CAD build for the part. Positions are in the model's coordinates, mm. Round coordinates to 2 decimals unless told otherwise and drop trailing zeros. Loops run counter-clockwise (first coordinate to the right, second up) from the corner with the lowest first, then second, coordinate; pieces in that order, holes last. Notation, with made-up numbers: (60.25, 50) -> (70.25, 50) arc R25 ccw to (70.25, 89) -> close; hole circle Ø10 at (8.5, 2.25). An arc over 180 degrees is marked (long way). Answer as CSV lines item,"result".
```python
from build123d import *

# Parameters (mm, degrees)
M2_5_TAPPED_HOLE1_D           = 2.05
M2_5_TAPPED_HOLE1_ON_FACE_2_D = 2.05


with BuildPart() as part:
    # Sketch1 → Revolve1 (revolve)
    with BuildSketch(Plane.XY, mode=Mode.PRIVATE) as revolve1_sk:
        Polygon((0, 7.5), (36.519586152, 14), (36.519586152, 16.526331), (-23.480413848, 16.526331), (-23.480413848, 12.526331), align=None)
    revolve(revolve1_sk.sketch.rotate(Axis((-21.926609295, 0, 0), (1, 0, 0)), 90), axis=Axis((-21.926609295, 0, 0), (1, 0, 0)))

    # M2.5 Tapped Hole1 (through all)
    with Locations(Plane(origin=(-20.480413848, 0, -16.526331), x_dir=(0, -1, 0), z_dir=(0, 0, -1))):
        with Locations((0, 0)):
            Hole(M2_5_TAPPED_HOLE1_D / 2)

    # M2.5 Tapped Hole1 on face 2 (through all)
    with Locations(Plane(origin=(-20.480413848, 16.526331, 0), x_dir=(0, 0, 1), z_dir=(0, 1, 0))):
        with Locations((0, 0)):
            Hole(M2_5_TAPPED_HOLE1_ON_FACE_2_D / 2)


solid = part.part
```
Q1. Slice it at D-D, the plane x = 9. Give the cut face in (y, z).
Results:
outline,"circle Ø33.05 at (0, 0); hole circle Ø18.2 at (0, 0)"
Q2. Probe L1, parallel to Z at x = 21.5, y = -3.5; L2, parallel to Z at x = -10.5, y = 6.5; L3, parallel to Y at x = -16, z = 5.5. List the from-to ranges inside material, lowest first. Write a range as [from, to].
Results:
L1,"[-16.15, -10.77], [10.77, 16.15]"
L2,"[-15.19, -7.26], [7.26, 15.19]"
L3,"[-15.58, -9.44], [9.44, 15.58]"
Q3. Slice it at A-A, the plane y = 0. Give the cut face in (x, z), and give its area (3 significant figures).
Results:
outline,"(-23.48, -16.53) -> (-21.51, -16.53) -> (-21.51, -12.1) -> (-23.48, -12.53) -> close; (-23.48, 12.53) -> (-21.51, 12.1) -> (-21.51, 16.53) -> (-23.48, 16.53) -> close; (-19.46, -16.53) -> (36.52, -16.53) -> (36.52, -14) -> (0, -7.5) -> (-19.46, -11.66) -> close; (-19.46, 11.66) -> (0, 7.5) -> (36.52, 14) -> (36.52, 16.53) -> (-19.46, 16.53) -> close"
area,"709 mm2"
Q4. Drop flat-ended pins along their axis: pin 1 Ø6 at (x, y) = (25, 13) entering from +Z; pin 2 Ø8 at (x, y) = (0.5, 5) entering from +Z; pin 3 Ø1 at (y, z) = (-3, 6) entering from +X; pin 4 Ø6 at (x, z) = (-6, -9.5) entering from +Y. Give the stop position or say it passes through.
Results:
pin 1,"z = 13.16"
pin 2,"z = 16.5"
pin 3,"through"
pin 4,"y = 15.19"
Q5. Slice it at C-C, the plane x = -8. Give the cut face in (y, z).
Results:
outline,"circle Ø33.05 at (0, 0); hole circle Ø18.43 at (0, 0)"
Q6. Two-plate mould, pull along Y, no slides. Class faces 1 (the cylindrical face through (-19.48, -0.22, -14.06)), 2 (the flat face through (36.52, -4, 14)), 3 (the cylindrical face through (6.1, -4.964, 15.763)): pulls with the +Y half, pulls with the -Y half, needs draft (parallel to the pull), parting line crosses it, or undercut.
Results:
face 1,"undercut"
face 2,"needs draft"
face 3,"parting line crosses it"
